Verification items for the finished model (mm, model axes). Give positions to 0.01 mm unless a question says otherwise; leave off trailing zeros. Order: outer loops, then holes, each group sorted by start corner. A loop starts at its lowest first (then second) coordinate and runs counter-clockwise, first axis right, second up. Notation, with made-up numbers: (50.25, 67.25) - (65.25, 67.25) arc R9 ccw to (65.25, 76.25) - close; hole circle Ø6 at (63.25, 58). An arc over 180 degrees is marked (long way). Answer as a JSON object with one key per item and string values. Group by question number.
(1) Section check B-B (x = -664.5). Record the boundary of the cut face in (y, z).
(2) Thickness scan on line 1 (Y direction, x = -855, z = 2.05); line 2 (Y direction, x = -601, z = 1.75). Record the ranges inside material, lowest first.
(3) Section check C-C (x = -539). Record the boundary of the cut face in (y, z), then the cut area to 3 significant figures.
(4) Depth check by flat-ended pin: pin 1 Ø1 at (x, z) = (-847, 1) entering from -Y; pin 2 Ø1 at (x, y) = (-648, 52) entering from +Z; pin 3 Ø1 at (x, z) = (-850.5, 0.5) entering from -Y. Enter the tip coordinate at first touch or a pass-through.
```python
from build123d import *

# Parameters (mm, degrees)
BOSS_EXTRUDE1_DEPTH     = 2.54
CUT_EXTRUDE1_DEPTH      = 1
CUT_EXTRUDE1_DEPTH_BACK = 3.54
CUT_EXTRUDE2_DEPTH      = 7.62


with BuildPart() as part:
    # Sketch1 → Boss-Extrude1 (new body)
    with BuildSketch(Plane.XY):
        Polygon((-945.957227657, 86.137779906), (-945.969713578, 86.1172966), (-949.121092485, 86.403457059), (-949.65244679, 80.075727402), (-9.887238192, -5.25964904), (-6.723373364, -5.525326193), (0, -5.833733414), (152.4, -5.833733414), (152.4, 11.946266586), (139.7, 11.946266586), (139.7, 6.866266586), (136.525, 6.866266586), (136.525, 11.946266586), (95.25, 11.946266586), (95.25, 6.866266586), (92.075, 6.866266586), (92.075, 11.946266586), (79.375, 11.946266586), (79.375, 6.866266586), (76.2, 6.866266586), (76.2, 11.946266586), (69.85, 11.946266586), (25.4, 19.566266586), (19.05, 19.566266586), (19.05, 14.486266586), (15.875, 14.486266586), (15.875, 19.566266586), (3.175, 19.566266586), (3.175, 13.216266586), (0, 13.216266586), (0, 19.566266586), (-1.98607431, 19.566266586), (-4.597956143, 19.785592432), (-5.129310448, 13.457862776), (-8.293175277, 13.723539928), (-7.761820971, 20.051269584), (-944.89858306, 98.744842179), align=None)
    extrude(amount=BOSS_EXTRUDE1_DEPTH)

    # Sketch2 → Cut-Extrude1 (cut, two sides)
    with BuildSketch(Plane.XY.offset(2.54)) as cut_extrude1_sk:
        Polygon((-867.4716203, 85.879017088), (-866.940953695, 92.198557139), (-870.104818523, 92.464234292), (-870.635482595, 86.144724398), align=None)
        Polygon((-788.501617399, 79.246962625), (-787.970887585, 85.567255411), (-791.134752413, 85.832932563), (-791.665479694, 79.512669935), align=None)
        Polygon((-709.531614498, 72.614908162), (-709.000821475, 78.935953682), (-712.164686303, 79.201630835), (-712.695476794, 72.880615473), align=None)
        Polygon((-630.561611597, 65.9828537), (-630.030755365, 72.304651954), (-633.194620194, 72.570329107), (-633.725473893, 66.24856101), align=None)
        Polygon((-551.591608696, 59.350799237), (-551.060689256, 65.673350226), (-554.224554084, 65.939027378), (-554.755470992, 59.616506547), align=None)
        Polygon((-472.621605795, 52.718744774), (-472.090623146, 59.042048497), (-475.254487974, 59.30772565), (-475.785468091, 52.984452084), align=None)
        Polygon((-393.651602894, 46.086690311), (-393.120557036, 52.410746769), (-396.284421864, 52.676423921), (-396.81546519, 46.352397622), align=None)
        Polygon((-314.681599993, 39.454635849), (-314.150490926, 45.77944504), (-317.314355754, 46.045122193), (-317.845462289, 39.720343159), align=None)
        Polygon((-235.711597092, 32.822581386), (-235.180424816, 39.148143312), (-238.344289645, 39.413820465), (-238.875459388, 33.088288696), align=None)
        Polygon((-156.741594191, 26.190526923), (-156.210358707, 32.516841584), (-159.374223535, 32.782518736), (-159.905456487, 26.456234233), align=None)
        Polygon((-77.240292597, 25.885539855), (-80.404157425, 26.151217008), (-80.935453586, 19.824179771), (-77.77159129, 19.55847246), align=None)
    extrude(amount=CUT_EXTRUDE1_DEPTH, mode=Mode.SUBTRACT)
    extrude(cut_extrude1_sk.sketch, amount=-CUT_EXTRUDE1_DEPTH_BACK, mode=Mode.SUBTRACT)

    # Sketch3 → Cut-Extrude2 (cut)
    with BuildSketch(Plane.XY.offset(2.54)):
        Polygon((-434.187522505, 55.859236209), (-441.444486836, 50.074133547), (-431.803024179, 44.022577198), (-442.349656028, 39.171455119), (-433.014300591, 33.162402364), (148.326621663, -67.648294025), (201.247452175, 33.162402364), align=None)
    extrude(amount=-CUT_EXTRUDE2_DEPTH, mode=Mode.SUBTRACT)


solid = part.part
```
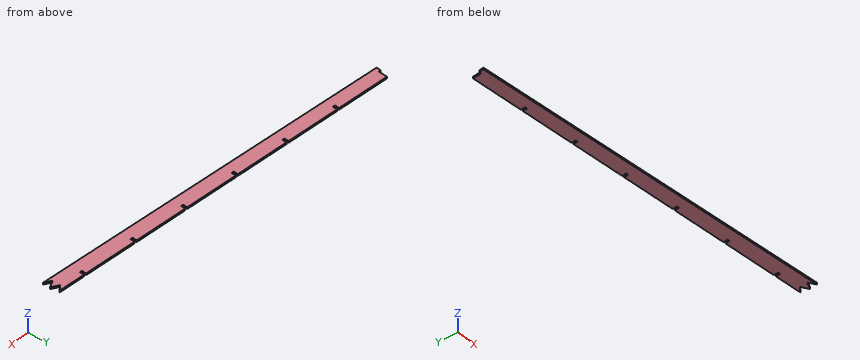
Solutions:
{
 "1": {"outline": "(54.18, 0) - (75.2, 0) - (75.2, 2.54) - (54.18, 2.54) - close"},
 "2": {"line 1": "y = 71.48 to 91.2", "line 2": "y = 48.42 to 69.87"},
 "3": {"outline": "(42.79, 0) - (64.66, 0) - (64.66, 2.54) - (42.79, 2.54) - close", "area": "55.6 mm2"},
 "4": {"pin 1": "stops at y = 70.71", "pin 2": "passes through", "pin 3": "stops at y = 71.03"}
}
